```python
from build123d import *

# Parameters (mm, degrees)
SKETCH_2_R      = 2.55
SKETCH_2_W      = 22
SKETCH_2_H      = 22
SKETCH_2_W_2    = 14
SKETCH_2_H_2    = 14
SKETCH_2_W_3    = 50
SKETCH_2_H_3    = 8
EXTRUDE_1_DEPTH = 5


with BuildPart() as part:
    # 草图2 → 凸台-拉伸1 (new body)
    with BuildSketch(Plane.XY):
        with BuildLine():
            Line((-130, -130), (130, -130))
            ThreePointArc((130, -130), (144.142135624, -124.142135624), (150, -110))
            Line((150, -110), (150, 10))
            ThreePointArc((150, 10), (144.142135624, 24.142135624), (130, 30))
            Line((130, 30), (-130, 30))
            ThreePointArc((-130, 30), (-144.142135624, 24.142135624), (-150, 10))
            Line((-150, 10), (-150, -110))
            ThreePointArc((-150, -110), (-144.142135624, -124.142135624), (-130, -130))
        make_face()
        with Locations((130, -110)):
            Circle(SKETCH_2_R, mode=Mode.SUBTRACT)
        with Locations((130, 10)):
            Circle(SKETCH_2_R, mode=Mode.SUBTRACT)
        with Locations((-130, -110)):
            Circle(SKETCH_2_R, mode=Mode.SUBTRACT)
        with Locations((-130, 10)):
            Circle(SKETCH_2_R, mode=Mode.SUBTRACT)
        with Locations((-61, -50)):
            Rectangle(SKETCH_2_W, SKETCH_2_H, mode=Mode.SUBTRACT)
        with Locations((-26, -50)):
            Rectangle(SKETCH_2_W, SKETCH_2_H, mode=Mode.SUBTRACT)
        with Locations((26, -50)):
            Rectangle(SKETCH_2_W, SKETCH_2_H, mode=Mode.SUBTRACT)
        with Locations((136, -87)):
            Rectangle(SKETCH_2_W_2, SKETCH_2_H_2, mode=Mode.SUBTRACT)
        with Locations((136, -13)):
            Rectangle(SKETCH_2_W_2, SKETCH_2_H_2, mode=Mode.SUBTRACT)
        Rectangle(SKETCH_2_W_3, SKETCH_2_H_3, mode=Mode.SUBTRACT)
        with Locations((-136, -87)):
            Rectangle(SKETCH_2_W_2, SKETCH_2_H_2, mode=Mode.SUBTRACT)
        with Locations((-136, -13)):
            Rectangle(SKETCH_2_W_2, SKETCH_2_H_2, mode=Mode.SUBTRACT)
        with Locations((-96, -50)):
            Rectangle(SKETCH_2_W, SKETCH_2_H, mode=Mode.SUBTRACT)
        with Locations((61, -50)):
            Rectangle(SKETCH_2_W, SKETCH_2_H, mode=Mode.SUBTRACT)
        with Locations((96, -50)):
            Rectangle(SKETCH_2_W, SKETCH_2_H, mode=Mode.SUBTRACT)
    extrude(amount=EXTRUDE_1_DEPTH)


solid = part.part
```
Can you work these out from the model? Positions are in its coordinate system, mm. Give positions to 0.01 mm unless a question says otherwise; leave off trailing zeros. Order: outer loops, then holes, each group sorted by start corner. A loop starts at its lowest first (then second) coordinate and runs counter-clockwise, first axis right, second up. Notation, with made-up numbers: M 13.25,85.5 L 36.25,85.5 A27 cw 36.25,122.5 Z; hole C 73.5,45 d7. An arc over 180 degrees is marked long. Write item = value, one per line. Start each with the question number.
Q1. Will these pins go through, and if not, where does the flat tip stop? pin 1 Ø1.5 at (x, z) = (137, 2) entering from -Y; pin 2 Ø2.5 at (x, z) = (-138.5, 2) entering from +Y.
Q2. I need wall thicknesses on probe 1 along Y at (x, z) = (-130, 3.6); probe 2 along X at (y, z) = (12, 3.5); probe 3 along Y at (x, z) = (66, 3.1). Which ranges of each line are inside material? Lowest first, please. Write a range as [from, to].
Q3. Suppose I cut it at A-A (x = 104). Write out the boundary of the cut face in (y, z), plus the area to 3 significant figures.
Q4. Suppose I cut it at B-B (z = 4). Count the separate pieces of the cut face and the enclosed holes in it, plus the area to 3 significant figures.
Q5. We'd pull the mould along Y, two halves only. Please class faces 1 (the cylindrical face through (-143.986, 24.297, 2.465)), 2 (the flat face through (-2, -49, 5)), 3 (the cylindrical face through (-144.297, -123.986, 2.465)): pulls with the +Y half, pulls with the -Y half, needs draft (parallel to the pull), parting line crosses it, or undercut.
Check result:
q1.pin_1 = -129
q1.pin_2 = 28.64
q2.probe_1 = [-130, -112.55], [-107.45, -94], [-80, -20], [-6, 7.45], [12.55, 30]
q2.probe_2 = [-149.9, -131.58], [-128.42, 128.42], [131.58, 149.9]
q2.probe_3 = [-130, -61], [-39, 30]
q3.outline = M -130,0 L -61,0 L -61,5 L -130,5 Z; M -39,0 L 30,0 L 30,5 L -39,5 Z
q3.area = 690 mm2
q4.separate_pieces = 1
q4.enclosed_holes = 15
q4.area = 43,500 mm2
q5.face_1 = pulls with the +Y half
q5.face_2 = needs draft
q5.face_3 = pulls with the -Y half
